Input: dimensioned drawing with shaded views. Units: mm. Origin: part minimum x, y, z. Give positions to 0.01 mm unless a question says otherwise; leave off trailing zeros. Order: outer loops, then holes, each group sorted by start corner. A loop starts at its lowest first (then second) coordinate and runs counter-clockwise, first axis right, second up.
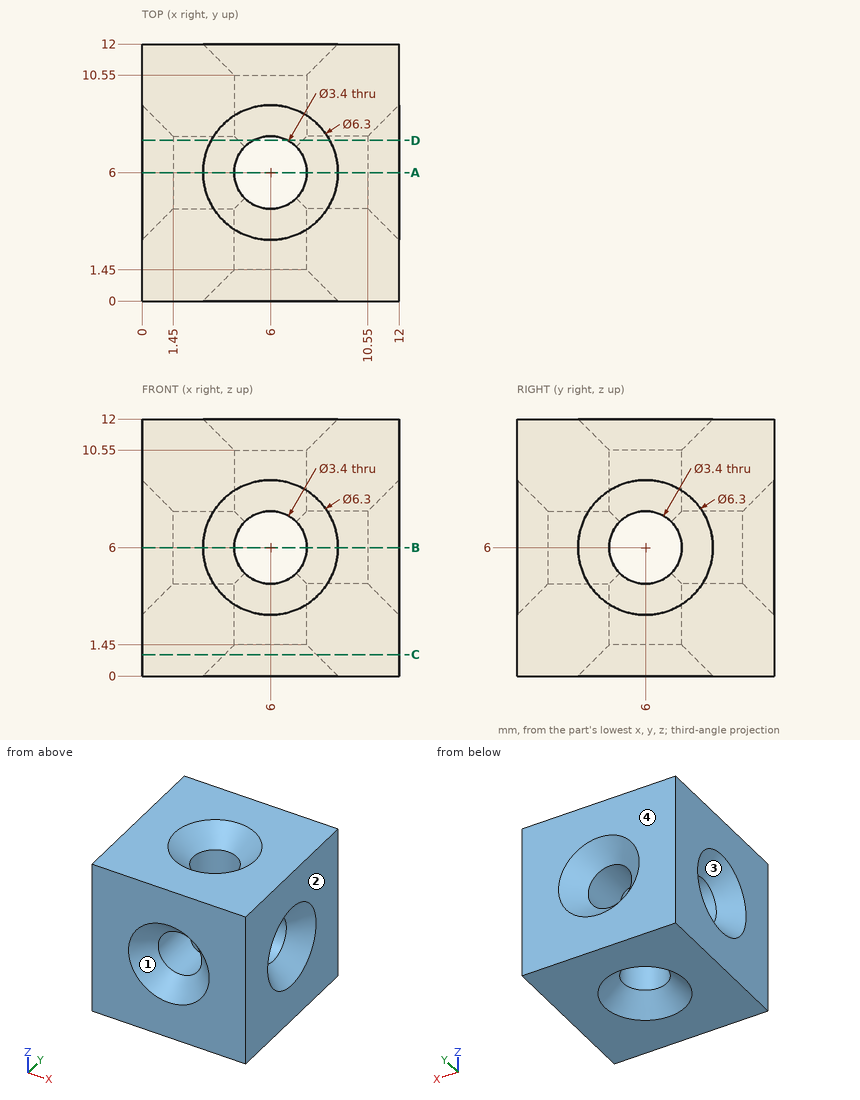
1) Pin query (flat end, axial travel): pin 1 (2 mm diameter, centred on x = 5.5, y = 3.5, fed in from +Z); pin 2 (2 mm diameter, centred on x = 6, y = 6, fed in from +Z); pin 3 (4.5 mm diameter, centred on y = 6, z = 6, fed in from -X); pin 4 (4.5 mm diameter, centred on x = 6, z = 6, fed in from +Y). Return the tip coordinate at first contact, or that it passes through.
Report:
pin 1: stops at z = 12
pin 2: passes through
pin 3: stops at x = 0.9
pin 4: stops at y = 11.1
2) Material intervals for L1, parallel to Y at x = 4.5, z = 5; L2, parallel to Z at x = 6, y = 9.6; L3, parallel to Z at x = 5.5, y = 3.75, sorted ascending.
Report:
L1: y = 1.35 to 4.63, 7.37 to 10.65
L2: z = 0 to 4.3, 7.7 to 12
L3: z = 0.85 to 4.38, 7.62 to 11.15
3) Section query C-C, the plane z = 1. Return the cut outline in (x, y).
Report:
outline: (0, 0) - (12, 0) - (12, 12) - (0, 12) - close; hole circle Ø4.3 at (6, 6)
4) Draft query along Y for the marked faces 1, 2, 3 and 4. Return one class per face: +Y half, -Y half, draft (parallel to the pull), parting line (faces both ways), or undercut.
Report:
face 1: -Y half
face 2: draft
face 3: undercut
face 4: +Y half
5) Section query D-D, the plane y = 7.5. Count the separate pieces of the cut face and the enclosed holes in it, and give its area (3 significant figures).
Report:
separate pieces: 4
enclosed holes: 0
area: 94.6 mm2
6) Section query A-A, the plane y = 6. Return the cut outline in (x, z), and give its area (4 significant figures).
Report:
outline: (0, 0) - (2.85, 0) - (4.3, 1.45) - (4.3, 4.3) - (1.45, 4.3) - (0, 2.85) - close; (0, 9.15) - (1.45, 7.7) - (4.3, 7.7) - (4.3, 10.55) - (2.85, 12) - (0, 12) - close; (7.7, 1.45) - (9.15, 0) - (12, 0) - (12, 2.85) - (10.55, 4.3) - (7.7, 4.3) - close; (7.7, 7.7) - (10.55, 7.7) - (12, 9.15) - (12, 12) - (9.15, 12) - (7.7, 10.55) - close
area: 65.55 mm2
